Part model, mm, in its own coordinate system. Face numbers are marked on the shaded views. Give positions to 0.01 mm unless a question says otherwise; leave off trailing zeros. Write each loop counter-clockwise with the first axis right and the second up, starting at its lowest first coordinate (ties: lowest second). Pieces come first, ordered by that corner, then holes.
from build123d import *

# Parameters (mm, degrees)
F0_R     = 10.9855
F1_DEPTH = 6.985


with BuildPart() as f1:
    # F0 (on Top) → F1 (new body)
    with BuildSketch(Plane.XY):
        with BuildLine():
            ThreePointArc((-21.668307594, 0), (-18.2243869403, 4.4968425779), (-13.8658100212, 8.1141606286))
            ThreePointArc((-13.8658100212, 8.1141606286), (-16.0655, 0), (-13.8658100212, -8.1141606286))
            ThreePointArc((-13.8658100212, -8.1141606286), (-9.0413202093, -13.2798651771), (-2.4667114241, -15.875))
            ThreePointArc((-2.4667114241, -15.875), (-2.6336178966, -15.9018345849), (-2.8002327647, -15.9304239401))
            ThreePointArc((-2.8002327647, -15.9304239401), (-12.5689671865, -21.743934134), (-16.044699379, -32.5672588867))
            ThreePointArc((-16.044699379, -32.5672588867), (-15.6474770652, -35.3909822497), (-14.75729617, -38.1))
            ThreePointArc((-14.75729617, -38.1), (0, -47.8155), (14.75729617, -38.1))
            ThreePointArc((14.75729617, -38.1), (15.6474770652, -35.3909822497), (16.044699379, -32.5672588867))
            ThreePointArc((16.044699379, -32.5672588867), (12.5689671865, -21.743934134), (2.8002327647, -15.9304239401))
            ThreePointArc((2.8002327647, -15.9304239401), (2.6336178966, -15.9018345849), (2.4667114241, -15.875))
            ThreePointArc((2.4667114241, -15.875), (9.0413202093, -13.2798651771), (13.8658100212, -8.1141606286))
            ThreePointArc((13.8658100212, -8.1141606286), (16.0655, 0), (13.8658100212, 8.1141606286))
            ThreePointArc((13.8658100212, 8.1141606286), (18.2243869403, 4.4968425779), (21.668307594, 0))
            ThreePointArc((21.668307594, 0), (22.7248224192, 1.9453544448), (23.6071191459, 3.9756696857))
            ThreePointArc((23.6071191459, 3.9756696857), (14.4936570973, 12.1982197779), (2.8002327647, 15.9304239401))
            ThreePointArc((2.8002327647, 15.9304239401), (12.5689671865, 21.743934134), (16.044699379, 32.5672588867))
            ThreePointArc((16.044699379, 32.5672588867), (15.6474770652, 35.3909822497), (14.75729617, 38.1))
            ThreePointArc((14.75729617, 38.1), (0, 47.8155), (-14.75729617, 38.1))
            ThreePointArc((-14.75729617, 38.1), (-15.6474770652, 35.3909822497), (-16.044699379, 32.5672588867))
            ThreePointArc((-16.044699379, 32.5672588867), (-12.5689671865, 21.743934134), (-2.8002327647, 15.9304239401))
            ThreePointArc((-2.8002327647, 15.9304239401), (-14.4936570973, 12.1982197779), (-23.6071191459, 3.9756696857))
            ThreePointArc((-23.6071191459, 3.9756696857), (-22.7248224192, 1.9453544448), (-21.668307594, 0))
        make_face()
        with Locations((0, -31.75)):
            Circle(F0_R, mode=Mode.SUBTRACT)
        Circle(F0_R, mode=Mode.SUBTRACT)
        with Locations((0, 31.75)):
            Circle(F0_R, mode=Mode.SUBTRACT)
        with BuildLine():
            ThreePointArc((-23.6071191459, -3.9756696857), (-22.7248224192, -1.9453544448), (-21.668307594, 0))
            ThreePointArc((-21.668307594, 0), (-22.7248224192, 1.9453544448), (-23.6071191459, 3.9756696857))
            ThreePointArc((-23.6071191459, 3.9756696857), (-24.8896850265, 2.0359533325), (-26.013236893, 0))
            ThreePointArc((-26.013236893, 0), (-24.8896850265, -2.0359533325), (-23.6071191459, -3.9756696857))
        make_face()
        with BuildLine():
            ThreePointArc((-26.013236893, 0), (-24.8896850265, 2.0359533325), (-23.6071191459, 3.9756696857))
            ThreePointArc((-23.6071191459, 3.9756696857), (-24.4425125824, 19.4925468905), (-16.044699379, 32.5672588867))
            ThreePointArc((-16.044699379, 32.5672588867), (-15.6474770652, 35.3909822497), (-14.75729617, 38.1))
            ThreePointArc((-14.75729617, 38.1), (-27.9009245646, 21.2703622392), (-26.013236893, 0))
        make_face()
        with BuildLine():
            ThreePointArc((-16.044699379, -32.5672588867), (-24.4425125824, -19.4925468905), (-23.6071191459, -3.9756696857))
            ThreePointArc((-23.6071191459, -3.9756696857), (-24.8896850265, -2.0359533325), (-26.013236893, 0))
            ThreePointArc((-26.013236893, 0), (-27.9009245646, -21.2703622392), (-14.75729617, -38.1))
            ThreePointArc((-14.75729617, -38.1), (-15.6474770652, -35.3909822497), (-16.044699379, -32.5672588867))
        make_face()
        with BuildLine():
            ThreePointArc((26.013236893, 0), (27.9009245646, 21.2703622392), (14.75729617, 38.1))
            ThreePointArc((14.75729617, 38.1), (15.6474770652, 35.3909822497), (16.044699379, 32.5672588867))
            ThreePointArc((16.044699379, 32.5672588867), (24.4425125824, 19.4925468905), (23.6071191459, 3.9756696857))
            ThreePointArc((23.6071191459, 3.9756696857), (24.8896850265, 2.0359533325), (26.013236893, 0))
        make_face()
        with BuildLine():
            ThreePointArc((16.044699379, -32.5672588867), (15.6474770652, -35.3909822497), (14.75729617, -38.1))
            ThreePointArc((14.75729617, -38.1), (27.9009245646, -21.2703622392), (26.013236893, 0))
            ThreePointArc((26.013236893, 0), (24.8896850265, -2.0359533325), (23.6071191459, -3.9756696857))
            ThreePointArc((23.6071191459, -3.9756696857), (24.4425125824, -19.4925468905), (16.044699379, -32.5672588867))
        make_face()
        with BuildLine():
            ThreePointArc((23.6071191459, -3.9756696857), (24.8896850265, -2.0359533325), (26.013236893, 0))
            ThreePointArc((26.013236893, 0), (24.8896850265, 2.0359533325), (23.6071191459, 3.9756696857))
            ThreePointArc((23.6071191459, 3.9756696857), (22.7248224192, 1.9453544448), (21.668307594, 0))
            ThreePointArc((21.668307594, 0), (22.7248224192, -1.9453544448), (23.6071191459, -3.9756696857))
        make_face()
        with BuildLine():
            ThreePointArc((-2.4667114241, -15.875), (-9.0413202093, -13.2798651771), (-13.8658100212, -8.1141606286))
            ThreePointArc((-13.8658100212, -8.1141606286), (-18.2243869403, -4.4968425779), (-21.668307594, 0))
            ThreePointArc((-21.668307594, 0), (-22.7248224192, -1.9453544448), (-23.6071191459, -3.9756696857))
            ThreePointArc((-23.6071191459, -3.9756696857), (-14.4936570973, -12.1982197779), (-2.8002327647, -15.9304239401))
            ThreePointArc((-2.8002327647, -15.9304239401), (-2.6336178966, -15.9018345849), (-2.4667114241, -15.875))
        make_face()
        with BuildLine():
            ThreePointArc((2.8002327647, -15.9304239401), (14.4936570973, -12.1982197779), (23.6071191459, -3.9756696857))
            ThreePointArc((23.6071191459, -3.9756696857), (22.7248224192, -1.9453544448), (21.668307594, 0))
            ThreePointArc((21.668307594, 0), (18.2243869403, -4.4968425779), (13.8658100212, -8.1141606286))
            ThreePointArc((13.8658100212, -8.1141606286), (9.0413202093, -13.2798651771), (2.4667114241, -15.875))
            ThreePointArc((2.4667114241, -15.875), (2.6336178966, -15.9018345849), (2.8002327647, -15.9304239401))
        make_face()
    extrude(amount=F1_DEPTH)


solid = f1.part
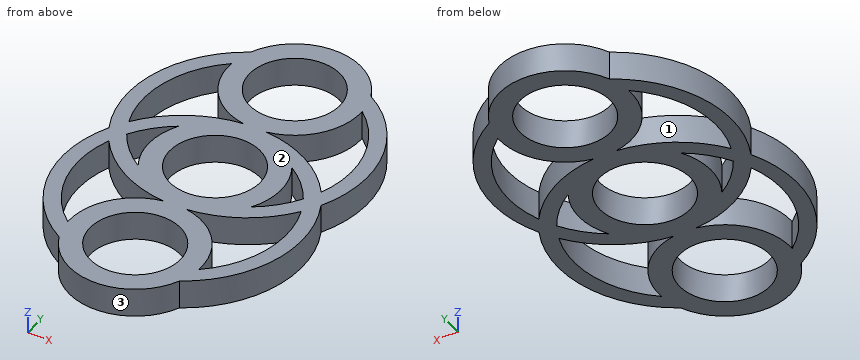
1) Saw through at B-B (y = -40.5). Write the cut outline in (x, z) (3 decimals).
Check result:
outline: (-13.474, 0) - (-6.642, 0) - (-6.642, 6.985) - (-13.474, 6.985) - close; (6.642, 0) - (13.474, 0) - (13.474, 6.985) - (6.642, 6.985) - close
2) Saw through at D-D (x = 6). Write the cut outline in (y, z) (3 decimals).
Check result:
outline: (-46.653, 0) - (-40.952, 0) - (-40.952, 6.985) - (-46.653, 6.985) - close; (-22.548, 0) - (-16.847, 0) - (-16.847, 6.985) - (-22.548, 6.985) - close; (-15.44, 0) - (-9.202, 0) - (-9.202, 6.985) - (-15.44, 6.985) - close; (9.202, 0) - (15.44, 0) - (15.44, 6.985) - (9.202, 6.985) - close; (16.847, 0) - (22.548, 0) - (22.548, 6.985) - (16.847, 6.985) - close; (40.952, 0) - (46.653, 0) - (46.653, 6.985) - (40.952, 6.985) - close
3) Saw through at C-C (z = 2). State how many separate pieces and enclosed holes the cut face has, and give its area (3 significant figures).
Check result:
separate pieces: 1
enclosed holes: 9
area: 2,150 mm2
4) Drill centre lines: L1, parallel to Y at x = 23, z = 5.75; L2, parallel to Y at x = 13, z = 6.5; L3, parallel to Y at x = 10, z = 3.25. Where is each one in solid material? Low to high.
Check result:
L1: y = -30.84 to -23.53, -4.79 to 4.79, 23.53 to 30.84
L2: y = -41.19 to -22.31, -13 to 13, 22.31 to 41.19
L3: y = -44.32 to -36.3, -27.2 to -19.18, -14.29 to -4.55, 4.55 to 14.29, 19.18 to 27.2, 36.3 to 44.32
5) Mould opens along Y. For the marked faces 1, 2 and 3 say: +Y half, -Y half, draft (parallel to the pull), parting line (faces both ways), or undercut.
Check result:
face 1: undercut
face 2: draft
face 3: -Y half
6) Flat gauge pins, fed straight in: P1, Ø1.5, axis at x = 14.5, z = 3.5, coming from the +Y side; P2, Ø1.5, axis at x = -6, z = 2.5, coming from the +Y side; P3, Ø1.5, axis at x = 7, z = 5, coming from the -Y side. Where does each tip first touch, or does it go through?
Check result:
P1: stops at y = 40.06
P2: stops at y = 46.93
P3: stops at y = -46.55
7) Saw through at A-A (x = 0). Write the cut outline in (y, z) (1 decimal).
Check result:
outline: (-47.8, 0) - (-42.7, 0) - (-42.7, 7) - (-47.8, 7) - close; (-20.8, 0) - (-11, 0) - (-11, 7) - (-20.8, 7) - close; (11, 0) - (20.8, 0) - (20.8, 7) - (11, 7) - close; (42.7, 0) - (47.8, 0) - (47.8, 7) - (42.7, 7) - close
